Verification items for the finished model (mm, model axes). A direction names the side the tool comes from. Coordinates: 2 decimals unless noted, no trailing zeros. Order: outer loops, then holes, each group sorted by start corner. A loop starts at its lowest first (then second) coordinate and runs counter-clockwise, first axis right, second up.
Q1. Thickness scan on line 1 (X direction, y = 1, z = 4.5); line 2 (Z direction, x = -12.5, y = 6.75). Record the ranges inside material, lowest first.
Q2. Cross-section at B-B, the plane z = 0. Record the boundary of the cut face in (x, y).
Q3. Set-up check for faces 1 (the flat face through (-18.5, 3, 0)), 2 (the cylindrical face through (-16, 2, 0)): record each of +Z, -Z, +X, -X, +Y, -Y from which the full face is reachable in a straight line by a thin tool's end or side.
Q4. Cross-section at A-A, the plane y = 8.25. Record the boundary of the cut face in (x, z), and give its area (3 significant figures).
Q5. Cross-section at C-C, the plane x = -15. Record the boundary of the cut face in (y, z).
Q6. Cross-section at D-D, the plane y = 3.5. Record the boundary of the cut face in (x, z).
from build123d import *

# Parameters (mm, degrees)
SKETCH1_W           = 27
SKETCH1_H           = 22.3
BOSS_EXTRUDE1_DEPTH = 9
SKETCH2_R           = 1.5
BOSS_EXTRUDE3_DEPTH = 5
FILLET1_R           = 2


with BuildPart() as part:
    # Sketch1 → Boss-Extrude1 (new body)
    with BuildSketch(Plane(origin=(0, 0, 0), x_dir=(1, 0, 0), z_dir=(0, 1, 0))):
        Rectangle(SKETCH1_W, SKETCH1_H)
    extrude(amount=BOSS_EXTRUDE1_DEPTH)

    # Sketch2 → Boss-Extrude3 (add)
    with BuildSketch(Plane.ZY.offset(13.5)):
        with Locations(Location((0, 3.5, 0), (0, 0, 180))):
            Circle(SKETCH2_R)
    extrude(amount=BOSS_EXTRUDE3_DEPTH)

    # Fillet1
    fillet1_edges = [part.edges().sort_by_distance(p)[0] for p in [
        (13.5, 4.5, 11.15),
        (-13.5, 4.5, 11.15),
        (-13.5, 4.5, -11.15),
        (13.5, 4.5, -11.15),
    ]]
    fillet(fillet1_edges, radius=FILLET1_R)


solid = part.part
Check values:
1. line 1: x = -13.5 to 13.5
1. line 2: z = -10.88 to 10.88
2. outline: (-18.5, 2) - (-13.5, 2) - (-13.5, 0) - (13.5, 0) - (13.5, 9) - (-13.5, 9) - (-13.5, 5) - (-18.5, 5) - close
3. face 1: +Z, -Z, -X, +Y, -Y
3. face 2: -X
4. outline: (-13.5, -9.15) arc R2 ccw to (-11.5, -11.15) - (11.5, -11.15) arc R2 ccw to (13.5, -9.15) - (13.5, 9.15) arc R2 ccw to (11.5, 11.15) - (-11.5, 11.15) arc R2 ccw to (-13.5, 9.15) - close
4. area: 599 mm2
5. outline: circle Ø3 at (3.5, 0)
6. outline: (-18.5, -1.5) - (-13.5, -1.5) - (-13.5, -9.15) arc R2 ccw to (-11.5, -11.15) - (11.5, -11.15) arc R2 ccw to (13.5, -9.15) - (13.5, 9.15) arc R2 ccw to (11.5, 11.15) - (-11.5, 11.15) arc R2 ccw to (-13.5, 9.15) - (-13.5, 1.5) - (-18.5, 1.5) - close
